```python
from build123d import *

# Parameters (mm, degrees)
CHAMFER1_SIZE  = 1.5
R1_RUNDING_R   = 1
SEKSKANT_DEPTH = 10


# Read off the part's stored shape, not the designer's step: Hul for sekskant
with BuildPart() as part:
    # Sketch1 → Base-Revolve (revolve)
    with BuildSketch(Plane.XY):
        Polygon((-36, 0), (-36, 10), (-33, 10), (-31, 12), (0, 12), (0, 0), align=None)
    revolve(axis=Axis((2, 0, 0), (-1, 0, 0)))

    # Chamfer1
    chamfer1_edges = [part.edges().sort_by_distance(p)[0] for p in [
        (0, -12, 0),
    ]]
    chamfer(chamfer1_edges, length=CHAMFER1_SIZE)

    # R1 runding
    r1_runding_edges = [part.edges().sort_by_distance(p)[0] for p in [
        (-36, -10, 0),
    ]]
    fillet(r1_runding_edges, radius=R1_RUNDING_R)

    # Hul for sekskant outline → Hul for sekskant (revolve, cut)
    with BuildSketch(Plane.YX):
        Polygon((0, 0), (0, -13.802581857), (3, -12), (3, 0), align=None)
    revolve(axis=Axis((0, 0, 0), (1, 0, 0)), mode=Mode.SUBTRACT)

    # Sketch8 → Sekskant (cut)
    with BuildSketch(Plane(origin=(0, 0, 0), x_dir=(0, 0, -1), z_dir=(1, 0, 0))):
        Polygon((-3, -1.732050808), (0, -3.464101615), (3, -1.732050808), (3, 1.732050808), (0, 3.464101615), (-3, 1.732050808), align=None)
    extrude(amount=-SEKSKANT_DEPTH, mode=Mode.SUBTRACT)


solid = part.part
```
Part model, mm, in its own coordinate system. A direction names the side the tool comes from. Coordinates: 2 decimals unless noted, no trailing zeros. Order: outer loops, then holes, each group sorted by start corner. A loop starts at its lowest first (then second) coordinate and runs counter-clockwise, first axis right, second up. Notation, with made-up numbers: (-5.75, -23) - (52.25, -23) arc R20 cw to (52.25, -16) - close; hole circle Ø3 at (27, 27.5). An arc over 180 degrees is marked (long way). Return JSON: item names as keys, results as strings. Group by question number.
Item 1: Pull direction Z, two halves, no side cores. Call faces 4 (the face through (-36, 0, 0)), 5 (the face through (-16.04, -11.99, -0.53)), 6 (the face through (-5, 0, 3)), 7 (the face through (-5, 0, -3)): pulls with the +Z half, pulls with the -Z half, needs draft (parallel to the pull), parting line crosses it, or undercut.
Item 2: Cut at B-B (x = -15). List the corners of the cut face in (y, z), plus the area to 3 significant figures.
Item 3: Cut at A-A (x = -8). List the corners of the cut face in (y, z), plus the area to 3 significant figures.
Item 4: Drill centre lines: probe 1 along Y at (x, z) = (-10.8, 0); probe 2 along Z at (x, y) = (-3, 2). Where is each one in solid material? Low to high. Write a range as from..to.
Item 5: Pin check, flat tips, straight feed: pin 1 (1.2 mm diameter, centred on y = -0.5, z = -2, fed in from +X); pin 2 (1.5 mm diameter, centred on x = -10.5, z = -4, fed in from +Y); pin 3 (1.5 mm diameter, centred on x = -26.5, z = -1, fed in from -Y). Stop position of each tip, or through.
Item 6: Which spindle directions (+Z, -Z, +X, -X, +Y, -Y) get a long thin tool onto all of the face, cutting with end or side? Do faces 1 (the face through (0, 2.2, -2.5)), 2 (the face through (-33.99, -2.17, 9.76)), 3 (the face through (-10, -3.2, 0)). Say none if no direction does.
Check values:
{
 "1": {"face 4": "needs draft", "face 5": "parting line crosses it", "face 6": "undercut", "face 7": "undercut"},
 "2": {"outline": "circle Ø24 at (0, 0)", "area": "452 mm2"},
 "3": {"outline": "circle Ø24 at (0, 0); hole (-3.46, 0) - (-1.73, -3) - (1.73, -3) - (3.46, 0) - (1.73, 3) - (-1.73, 3) - close", "area": "421 mm2"},
 "4": {"probe 1": "y = -12..-3, 3..12", "probe 2": "z = -11.83..-2.54, 2.54..11.83"},
 "5": {"pin 1": "stops at x = -12.2", "pin 2": "stops at y = 11.55", "pin 3": "stops at y = -12"},
 "6": {"face 1": "+Z, -Z, +X, +Y, -Y", "face 2": "-X", "face 3": "+X"}
}
